from build123d import *

# Parameters (mm, degrees)
BOSS_EXTRUDE1_DEPTH = 9
SKETCH2_W           = 1.8
SKETCH2_H           = 1.1
CUT_EXTRUDE1_DEPTH  = 24.178653973
SKETCH3_W           = 1.8
SKETCH3_H           = 1.1
CUT_EXTRUDE2_DEPTH  = 7


with BuildPart() as part:
    # Sketch1 → Boss-Extrude1 (new body)
    with BuildSketch(Plane.YZ):
        with BuildLine():
            Line((-15, -7.5), (15, -7.5))
            ThreePointArc((15, -7.5), (18.535533906, -6.035533906), (20, -2.5))
            Line((20, -2.5), (20, 2.5))
            ThreePointArc((20, 2.5), (18.535533906, 6.035533906), (15, 7.5))
            Line((15, 7.5), (-15, 7.5))
            ThreePointArc((-15, 7.5), (-18.535533906, 6.035533906), (-20, 2.5))
            Line((-20, 2.5), (-20, -2.5))
            ThreePointArc((-20, -2.5), (-18.535533906, -6.035533906), (-15, -7.5))
        make_face()
    extrude(amount=BOSS_EXTRUDE1_DEPTH)

    # Sketch2 → Cut-Extrude1 (cut, through all)
    with BuildSketch(Plane.YZ.offset(9)):
        with Locations((-12.25, 3.05)):
            Rectangle(SKETCH2_W, SKETCH2_H)
        with Locations((-15.75, 3.05)):
            Rectangle(SKETCH2_W, SKETCH2_H)
        with Locations((-8.75, 3.05)):
            Rectangle(SKETCH2_W, SKETCH2_H)
        with Locations((-5.25, 3.05)):
            Rectangle(SKETCH2_W, SKETCH2_H)
        with Locations((-1.75, 3.05)):
            Rectangle(SKETCH2_W, SKETCH2_H)
        with Locations((1.75, 3.05)):
            Rectangle(SKETCH2_W, SKETCH2_H)
        with Locations((5.25, 3.05)):
            Rectangle(SKETCH2_W, SKETCH2_H)
        with Locations((8.75, 3.05)):
            Rectangle(SKETCH2_W, SKETCH2_H)
        with Locations((12.25, 3.05)):
            Rectangle(SKETCH2_W, SKETCH2_H)
        with Locations((15.75, 3.05)):
            Rectangle(SKETCH2_W, SKETCH2_H)
        with Locations((-12.25, -3.05)):
            Rectangle(SKETCH2_W, SKETCH2_H)
        with Locations((-8.75, -3.05)):
            Rectangle(SKETCH2_W, SKETCH2_H)
        with Locations((-5.25, -3.05)):
            Rectangle(SKETCH2_W, SKETCH2_H)
        with Locations((-1.75, -3.05)):
            Rectangle(SKETCH2_W, SKETCH2_H)
        with Locations((1.75, -3.05)):
            Rectangle(SKETCH2_W, SKETCH2_H)
        with Locations((5.25, -3.05)):
            Rectangle(SKETCH2_W, SKETCH2_H)
        with Locations((8.75, -3.05)):
            Rectangle(SKETCH2_W, SKETCH2_H)
        with Locations((12.25, -3.05)):
            Rectangle(SKETCH2_W, SKETCH2_H)
        with Locations((15.75, -3.05)):
            Rectangle(SKETCH2_W, SKETCH2_H)
        with Locations((-15.75, -3.05)):
            Rectangle(SKETCH2_W, SKETCH2_H)
    extrude(amount=-CUT_EXTRUDE1_DEPTH, mode=Mode.SUBTRACT)

    # Sketch3 → Cut-Extrude2 (cut)
    with BuildSketch(Plane(origin=(0, 0, 0), x_dir=(0, -1, 0), z_dir=(-1, 0, 0))):
        with Locations((-15.75, 1.95)):
            Rectangle(SKETCH3_W, SKETCH3_H)
        with Locations((-12.25, 1.95)):
            Rectangle(SKETCH3_W, SKETCH3_H)
        with Locations((-8.75, 1.95)):
            Rectangle(SKETCH3_W, SKETCH3_H)
        with Locations((-5.25, 1.95)):
            Rectangle(SKETCH3_W, SKETCH3_H)
        with Locations((-1.75, 1.95)):
            Rectangle(SKETCH3_W, SKETCH3_H)
        with Locations((1.75, 1.95)):
            Rectangle(SKETCH3_W, SKETCH3_H)
        with Locations((5.25, 1.95)):
            Rectangle(SKETCH3_W, SKETCH3_H)
        with Locations((8.75, 1.95)):
            Rectangle(SKETCH3_W, SKETCH3_H)
        with Locations((12.25, 1.95)):
            Rectangle(SKETCH3_W, SKETCH3_H)
        with Locations((15.75, 1.95)):
            Rectangle(SKETCH3_W, SKETCH3_H)
        with Locations((-15.75, -4.15)):
            Rectangle(SKETCH3_W, SKETCH3_H)
        with Locations((-12.25, -4.15)):
            Rectangle(SKETCH3_W, SKETCH3_H)
        with Locations((-8.75, -4.15)):
            Rectangle(SKETCH3_W, SKETCH3_H)
        with Locations((-5.25, -4.15)):
            Rectangle(SKETCH3_W, SKETCH3_H)
        with Locations((-1.75, -4.15)):
            Rectangle(SKETCH3_W, SKETCH3_H)
        with Locations((1.75, -4.15)):
            Rectangle(SKETCH3_W, SKETCH3_H)
        with Locations((5.25, -4.15)):
            Rectangle(SKETCH3_W, SKETCH3_H)
        with Locations((8.75, -4.15)):
            Rectangle(SKETCH3_W, SKETCH3_H)
        with Locations((12.25, -4.15)):
            Rectangle(SKETCH3_W, SKETCH3_H)
        with Locations((15.75, -4.15)):
            Rectangle(SKETCH3_W, SKETCH3_H)
    extrude(amount=-CUT_EXTRUDE2_DEPTH, mode=Mode.SUBTRACT)


solid = part.part
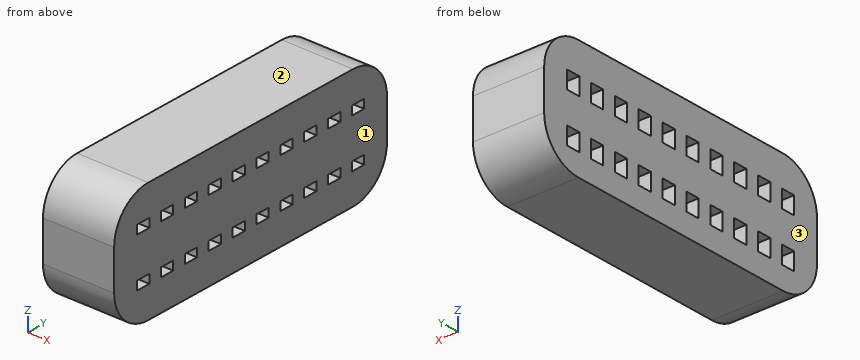
Geometry: final body of the model. Coordinates: model frame, mm. Face numbers are marked on the shaded views. Round coordinates to 2 decimals unless told otherwise and drop trailing zeros. Loops run counter-clockwise (first coordinate to the right, second up) from the corner with the lowest first, then second, coordinate; pieces in that order, holes last. Notation, with made-up numbers: M -31.5,16.5 L -16.5,16.5 A25 ccw -16.5,38.5 Z; hole C -31.5,-39 d4. An arc over 180 degrees is marked long. Put each result on its own line as item: value. Start each with the question number.
(1) Section query C-C (z = -5.5). Return loops of the section in (x, y).
(2) Section query A-A (y = -2). Return loops of the section in (x, z), then the cut area to 3 significant figures.
(3) Material intervals for line 1 along Z through (x, y) = (7.75, 1.5); line 2 along Z through (x, y) = (1.25, 1); line 3 along X through (y, z) = (-15, 1.5), sorted ascending. Write a range as [from, to].
(4) Section query B-B (x = 8.5). State how many separate pieces and enclosed holes the cut face has, then the cut area to 3 significant figures.
(5) Contact query for flat-ended pins moving along their axis: pin 1 Ø0.5 at (x, y) = (6.5, -15.5) entering from -Z; pin 2 Ø0.9 at (y, z) = (1.5, 2) entering from -X; pin 3 Ø1.1 at (x, z) = (5.5, -3.5) entering from +Y. Output: stop coordinate, or through.
(6) Draft query along X for the marked faces 1, 2 and 3. Return one class per face: +X half, -X half, draft (parallel to the pull), parting line (faces both ways), or undercut.
Findings below:
1. outline: M 0,-19 L 9,-19 L 9,19 L 0,19 Z
2. outline: M 0,-7.5 L 9,-7.5 L 9,-3.6 L 7,-3.6 L 7,-4.7 L 0,-4.7 Z; M 0,-2.5 L 9,-2.5 L 9,2.5 L 7,2.5 L 7,1.4 L 0,1.4 Z; M 0,3.6 L 9,3.6 L 9,7.5 L 0,7.5 Z
2. area: 99.8 mm2
3. line 1: z = [-7.5, -3.6], [-2.5, 2.5], [3.6, 7.5]
3. line 2: z = [-7.5, -4.7], [-2.5, 1.4], [3.6, 7.5]
3. line 3: x = [7, 9]
4. separate pieces: 1
4. enclosed holes: 20
4. area: 539 mm2
5. pin 1: stops at z = -7.49
5. pin 2: stops at x = 7
5. pin 3: stops at y = 19.98
6. face 1: +X half
6. face 2: draft
6. face 3: -X half
